For this review, take the finished solid that the model builds, in its own axes (mm). Face numbers are marked on the shaded views. A direction names the side the tool comes from. Coordinates: 2 decimals unless noted, no trailing zeros. Write each loop counter-clockwise with the first axis right and the second up, starting at its lowest first coordinate (ties: lowest second). Pieces come first, ordered by that corner, then holes.
```python
from build123d import *

# Parameters (mm, degrees)
SKETCH_1_R          = 6
EXTRUDE_1_DEPTH     = 1.5
SKETCH_2_R          = 4
EXTRUDE_2_DEPTH     = 0.5
SKETCH_3_R          = 4.5
EXTRUDE_3_DEPTH     = 0.5
SKETCH_4_R          = 3.5
CUT_EXTRUDE_1_DEPTH = 0.5
SKETCH_8_R          = 1.75
EXTRUDE_5_DEPTH     = 2
SKETCH_9_R          = 2.25
CUT_EXTRUDE_3_DEPTH = 2.5
FILLET_1_R          = 0.5
SKETCH_5_R          = 1.2
CUT_EXTRUDE_2_DEPTH = 2.4


with BuildPart() as part:
    # ｽｹｯﾁ1 → ﾎﾞｽ - 押し出し1 (new body)
    with BuildSketch(Plane(origin=(0, 0, 0), x_dir=(1, 0, 0), z_dir=(0, 1, 0))):
        with Locations(Location((0, 0, 0), (0, 0, 270))):
            Circle(SKETCH_1_R)
    extrude(amount=EXTRUDE_1_DEPTH)

    # ｽｹｯﾁ2 → ﾎﾞｽ - 押し出し2 (add)
    with BuildSketch(Plane(origin=(0, 1.5, 0), x_dir=(1, 0, 0), z_dir=(0, 1, 0))):
        with Locations(Location((0, 0, 0), (0, 0, 270))):
            Circle(SKETCH_2_R)
    extrude(amount=EXTRUDE_2_DEPTH)

    # ｽｹｯﾁ3 → ﾎﾞｽ - 押し出し3 (add)
    with BuildSketch(Plane.XZ):
        with Locations(Location((0, 0, 0), (0, 0, 270))):
            Circle(SKETCH_3_R)
    extrude(amount=EXTRUDE_3_DEPTH)

    # ｽｹｯﾁ4 → ｶｯﾄ - 押し出し1 (cut)
    with BuildSketch(Plane.XZ.offset(0.5)):
        with Locations(Location((0, 0, 0), (0, 0, 270))):
            Circle(SKETCH_4_R)
    extrude(amount=-CUT_EXTRUDE_1_DEPTH, mode=Mode.SUBTRACT)

    # ｽｹｯﾁ8 → ﾎﾞｽ - 押し出し5 (add, symmetric)
    with BuildSketch(Plane.XY):
        with BuildLine():
            Line((-3.55, 2), (-3.55, 7.65))
            ThreePointArc((-3.55, 7.65), (0, 11.2), (3.55, 7.65))
            Line((3.55, 7.65), (3.55, 2))
            Line((3.55, 2), (-3.55, 2))
        make_face()
        with Locations((0, 7.65)):
            Circle(SKETCH_8_R, mode=Mode.SUBTRACT)
    extrude(amount=EXTRUDE_5_DEPTH, both=True)

    # ｽｹｯﾁ9 → ｶｯﾄ - 押し出し3 (cut)
    with BuildSketch(Plane.XY.offset(2)):
        with Locations((0, 7.65)):
            Circle(SKETCH_9_R)
    extrude(amount=-CUT_EXTRUDE_3_DEPTH, mode=Mode.SUBTRACT)

    # ﾌｨﾚｯﾄ1
    # the kernel refuses this fillet: 0.5 mm, written as the material it takes off along each edge
    with BuildSketch(Plane(origin=(3.55, 7.65, 2), x_dir=(-1, 0, 0), z_dir=(0, -1, 0)), Plane(origin=(-3.55, 2, 2), x_dir=(1, 0, 0), z_dir=(0, 1, 0)), Plane(origin=(-3.55, 2, -2), x_dir=(0, 0, 1), z_dir=(0, 1, 0))) as fillet_1_piece_1:
        with BuildLine():
            CenterArc((FILLET_1_R, FILLET_1_R), FILLET_1_R, 180, 90)
            Line((0, FILLET_1_R), (0, 0))
            Line((0, 0), (FILLET_1_R, 0))
        make_face()
    extrude(amount=5.65, mode=Mode.SUBTRACT)
    with BuildSketch(Plane(origin=(0, 7.65, 2), x_dir=(-1, 0, 0), z_dir=(0, -1, 0))) as fillet_1_piece_2:
        with BuildLine():
            CenterArc((3.55 - FILLET_1_R, FILLET_1_R), FILLET_1_R, 270, 90)
            Line((3.55, FILLET_1_R), (3.55, 0))
            Line((3.55, 0), (3.55 - FILLET_1_R, 0))
        make_face()
    revolve(axis=Axis((0, 7.65, 2), (0, 0, -1)), revolution_arc=180, mode=Mode.SUBTRACT)
    with BuildSketch(Plane(origin=(3.55, 7.65, -2), x_dir=(-1, 0, 0), z_dir=(0, -1, 0))) as fillet_1_piece_3:
        with BuildLine():
            CenterArc((FILLET_1_R, -FILLET_1_R), FILLET_1_R, 90, 90)
            Line((0, -FILLET_1_R), (0, 0))
            Line((0, 0), (FILLET_1_R, 0))
        make_face()
    extrude(amount=5.65, mode=Mode.SUBTRACT)
    with BuildSketch(Plane(origin=(0, 7.65, -2), x_dir=(-1, 0, 0), z_dir=(0, -1, 0))) as fillet_1_piece_4:
        with BuildLine():
            CenterArc((3.55 - FILLET_1_R, -FILLET_1_R), FILLET_1_R, 0, 90)
            Line((3.55, -FILLET_1_R), (3.55, 0))
            Line((3.55, 0), (3.55 - FILLET_1_R, 0))
        make_face()
    revolve(axis=Axis((0, 7.65, -2), (0, 0, -1)), revolution_arc=180, mode=Mode.SUBTRACT)

    # ｽｹｯﾁ5 → ｶｯﾄ - 押し出し2 (cut)
    with BuildSketch(Plane.XZ):
        with Locations(Location((0, 0, 0), (0, 0, 270))):
            Circle(SKETCH_5_R)
    extrude(amount=-CUT_EXTRUDE_2_DEPTH, mode=Mode.SUBTRACT)


solid = part.part
```
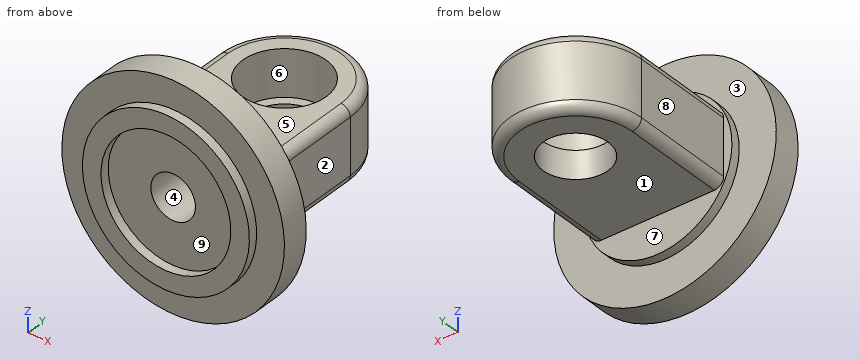
Q1. Tool access review of the marked faces 1, 2, 3, 4 and 5: name each direction out of +Z, -Z, +X, -X, +Y, -Y from which nothing blocks a thin tool from reaching the whole face with its end or side.
Ans:
face 1: -Z, +X, -X, +Y
face 2: +Z, -Z, +X, +Y
face 3: +Y
face 4: -Y
face 5: +Z, +X, -X, +Y
Q2. Clearance check with flat-ended pins moving along their axes: pin 1 Ø3 at (x, y) = (0, 5) entering from +Z; pin 2 Ø1.5 at (y, z) = (1.5, -4.5) entering from -X; pin 3 Ø0.9 at (y, z) = (4, 0.5) entering from -X; pin 4 Ø5 at (y, z) = (2, 0.5) entering from +X. State where each tip first meets the part, or that it passes through.
Ans:
pin 1: stops at z = 2
pin 2: stops at x = -4.68
pin 3: stops at x = -3.55
pin 4: stops at x = 6
Q3. Add section A-A (z = 0). State the section outline as (x, y) points, then the cut area to 3 significant figures.
Ans:
outline: (-6, 0) - (-4.5, 0) - (-4.5, -0.5) - (-3.5, -0.5) - (-3.5, 0) - (-1.2, 0) - (-1.2, 2.4) - (1.2, 2.4) - (1.2, 0) - (3.5, 0) - (3.5, -0.5) - (4.5, -0.5) - (4.5, 0) - (6, 0) - (6, 1.5) - (4, 1.5) - (4, 2) - (3.55, 2) - (3.55, 7.65) arc R3.55 ccw to (-3.55, 7.65) - (-3.55, 2) - (-4, 2) - (-4, 1.5) - (-6, 1.5) - close; hole circle Ø4.5 at (0, 7.65)
area: 61.2 mm2
Q4. Draft analysis for pull direction X (two halves, no side actions). For the marked faces 6, 7, 8 and 9, state which applies: +X half, -X half, draft (parallel to the pull), parting line (faces both ways), or undercut.
Ans:
face 6: undercut
face 7: draft
face 8: -X half
face 9: undercut
Q5. Add section D-D (z = 5.5). State the section outline as (x, y) points.
Ans:
outline: (-2.4, 0) - (2.4, 0) - (2.4, 1.5) - (-2.4, 1.5) - close
Q6. For probe 1 along X at (y, z) = (-0.05, 0); probe 2 along X at (y, z) = (0.7, 0); probe 3 along Y at (x, z) = (1.5, 3.75), list the stretches that pass through material, from the lowest coordinate up.
Ans:
probe 1: x = -4.5 to -3.5, 3.5 to 4.5
probe 2: x = -6 to -1.2, 1.2 to 6
probe 3: y = -0.5 to 1.5
Q7. Add section B-B (y = 3). State the section outline as (x, z) points, then the cut area to 3 significant figures.
Ans:
outline: (-3.55, -1.5) arc R0.5 ccw to (-3.05, -2) - (3.05, -2) arc R0.5 ccw to (3.55, -1.5) - (3.55, 1.5) arc R0.5 ccw to (3.05, 2) - (-3.05, 2) arc R0.5 ccw to (-3.55, 1.5) - close
area: 28.2 mm2
Q8. Add section C-C (z = 4.25). State the section outline as (x, y) points.
Ans:
outline: (-4.24, 0) - (-1.48, 0) - (-1.48, -0.5) - (1.48, -0.5) - (1.48, 0) - (4.24, 0) - (4.24, 1.5) - (-4.24, 1.5) - close
